Design review of the part built by this model. Coordinates are the model's own, in mm. Face numbers are marked on the shaded views. A direction names the side the tool comes from. Coordinates: 2 decimals unless noted, no trailing zeros. Write each loop counter-clockwise with the first axis right and the second up, starting at its lowest first coordinate (ties: lowest second). Pieces come first, ordered by that corner, then holes. Notation, with made-up numbers: (-10, 33.25) - (16, 33.25) arc R28 ccw to (16, 70.25) - close; hole circle Ø8 at (20, -35). An arc over 180 degrees is marked (long way). Use a Markdown table: item, result.
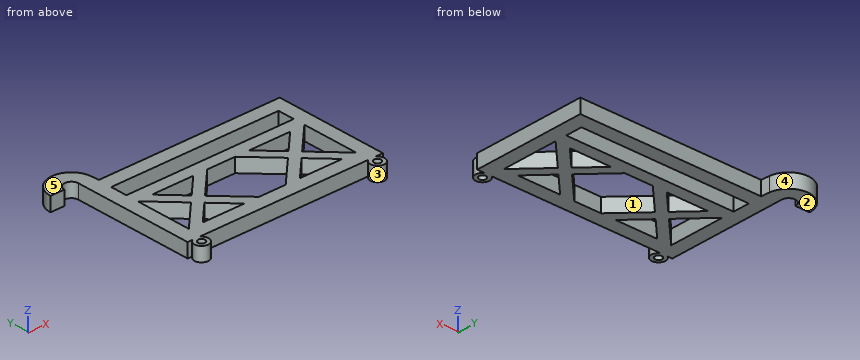
from build123d import *

# Parameters (mm, degrees)
SKETCH_R  = 0.5
SKETCH_W  = 24
SKETCH_H  = 2.370283
PAD_DEPTH = 2


with BuildPart() as part:
    # Sketch → Pad (new body)
    with BuildSketch(Plane.XY):
        with BuildLine():
            Line((-11.923108, 6.1), (14, 6.1))
            Line((14, 6.1), (14, -10))
            Line((12.932709, -10), (14, -10))
            ThreePointArc((11.932709, -10), (12.432709, -11.866025), (12.932709, -10))
            Line((-12.308759, -10), (11.932709, -10))
            ThreePointArc((-13.308759, -10), (-12.808759, -11.866025), (-12.308759, -10))
            Line((-14, -10), (-13.308759, -10))
            Line((-14, -10), (-14, 7.051026))
            ThreePointArc((-14, 7.051026), (-15.000062, 8.051026), (-16, 7.050903))
            Line((-18, 7.050903), (-16, 7.050903))
            ThreePointArc((-12.011962, 7.318663), (-15.134013, 10.048032), (-18, 7.050903))
            Line((-12.011962, 7.318663), (-11.923108, 6.1))
        make_face()
        with Locations((-12.808759, -10.866025)):
            Circle(SKETCH_R, mode=Mode.SUBTRACT)
        with Locations((12.432709, -10.866025)):
            Circle(SKETCH_R, mode=Mode.SUBTRACT)
        with Locations((0, 2.914858)):
            Rectangle(SKETCH_W, SKETCH_H, mode=Mode.SUBTRACT)
        Polygon((-12, -8), (-12, -0.037073), (-8.018537, -4.018537), align=None, mode=Mode.SUBTRACT)
        Polygon((-9.930922, 0), (-6.965461, -2.965461), (-4, 0), align=None, mode=Mode.SUBTRACT)
        Polygon((2, 0), (5.947956, -3.947956), (1.895912, -8), (-1.930922, -8), (-5.965461, -3.965461), (-2, 0), align=None, mode=Mode.SUBTRACT)
        Polygon((4, 0), (6.947956, -2.947956), (9.895912, 0), align=None, mode=Mode.SUBTRACT)
        Polygon((-10, -8), (-7.018537, -5.018537), (-4.037073, -8), align=None, mode=Mode.SUBTRACT)
        Polygon((3.930883, -8), (6.965441, -4.965441), (10, -8), align=None, mode=Mode.SUBTRACT)
        Polygon((7.965441, -3.965441), (12, 0.069117), (12, -8), align=None, mode=Mode.SUBTRACT)
    extrude(amount=PAD_DEPTH)


solid = part.part
(1) Machinability: for the marked faces 1 and 2, which of the approach directions +Z, -Z, +X, -X, +Y, -Y give a long, thin tool a straight path to every point of the face, cutting with its end or side? Answer none if there is none.
Determined:
| item | result |
|---|---|
| face 1 | +Z, -Z |
| face 2 | -Z, +X, -X, +Y, -Y |
(2) Draft analysis for pull direction Y (two halves, no side actions). For the marked faces 3, 4 and 5, state which applies: +Y half, -Y half, draft (parallel to the pull), parting line (faces both ways), or undercut.
Determined:
| item | result |
|---|---|
| face 3 | undercut |
| face 4 | +Y half |
| face 5 | draft |
(3) For pin 1 (1 mm diameter, centred on x = 0.5, z = 1, fed in from -Y); pin 2 (0.6 mm diameter, centred on y = -5, z = 1, fed in from -X); pin 3 (0.6 mm diameter, centred on x = -13.5, z = 0.5, fed in from -Y); pin 4 (1 mm diameter, centred on x = 7.5, y = -3, fed in from -Z), all flat-tipped, find the tip position at first contact; note any pin that passes through.
Determined:
| item | result |
|---|---|
| pin 1 | y = -10 |
| pin 2 | x = -14 |
| pin 3 | y = -11.79 |
| pin 4 | z = 0 |
(4) Take a section at A-A on x = -7.5. Write out the cut boundary in (y, z).
Determined:
| item | result |
|---|---|
| outline | (-10, 0) - (-8, 0) - (-8, 2) - (-10, 2) - close; (-5.5, 0) - (-2.43, 0) - (-2.43, 2) - (-5.5, 2) - close; (0, 0) - (1.73, 0) - (1.73, 2) - (0, 2) - close; (4.1, 0) - (6.1, 0) - (6.1, 2) - (4.1, 2) - close |
(5) Take a section at C-C on x = 7.5. Write out the cut boundary in (y, z).
Determined:
| item | result |
|---|---|
| outline | (-10, 0) - (-8, 0) - (-8, 2) - (-10, 2) - close; (-5.5, 0) - (-2.4, 0) - (-2.4, 2) - (-5.5, 2) - close; (0, 0) - (1.73, 0) - (1.73, 2) - (0, 2) - close; (4.1, 0) - (6.1, 0) - (6.1, 2) - (4.1, 2) - close |
(6) Take a section at D-D on y = -8.5. Write out the cut boundary in (x, z).
Determined:
| item | result |
|---|---|
| outline | (-14, 0) - (14, 0) - (14, 2) - (-14, 2) - close |
(7) For L1, parallel to Y at x = -1.5, z = 1.3; L2, parallel to Y at x = 6.5, z = 0.45; L3, parallel to Y at x = -9, z = 1.05, list the stretches that pass through material, from the lowest coordinate up. Write a range as from..to.
Determined:
| item | result |
|---|---|
| L1 | -10..-8, 0..1.73, 4.1..6.1 |
| L2 | -10..-8, -5.43..-2.5, 0..1.73, 4.1..6.1 |
| L3 | -10..-8, -7..-5, -3.04..-0.93, 0..1.73, 4.1..6.1 |
(8) Take a section at B-B on y = 3.75. Write out the cut boundary in (x, z), and give its area (3 significant figures).
Determined:
| item | result |
|---|---|
| outline | (-14, 0) - (-12, 0) - (-12, 2) - (-14, 2) - close; (12, 0) - (14, 0) - (14, 2) - (12, 2) - close |
| area | 8.00 mm2 |
